Source: CAD feature listing. Evaluate the final solid. Frame: model axes, mm. Round coordinates to 2 decimals unless told otherwise and drop trailing zeros. Loops run counter-clockwise (first coordinate to the right, second up) from the corner with the lowest first, then second, coordinate; pieces in that order, holes last. Notation, with made-up numbers: M -27,-14.5 L 2,-14.5 A24 cw 2,10.5 Z; hole C -34,43.25 d11. An arc over 180 degrees is marked long. Answer as a JSON object with one key per item and string values.
from build123d import *

# Parameters (mm, degrees)
SKETCH1_R             = 5.75
BOSS_EXTRUDE1_DEPTH   = 3
BOSS_EXTRUDE2_DEPTH   = 0.15
CIRPATTERN1_COUNT     = 2
SKETCH4_R             = 2.5
CUT_EXTRUDE1_DEPTH    = 7.0000001
FILLET1_R             = 0.5
CHAMFER1_SIZE         = 1
CHAMFER1_SIZE2        = 1.191753593
CHAMFER1_PART_2_SIZE  = 1
CHAMFER1_PART_2_SIZE2 = 1.191753593


with BuildPart() as part:
    # Sketch1 → Boss-Extrude1 (new body, symmetric)
    with BuildSketch(Plane(origin=(0, 0, 0), x_dir=(1, 0, 0), z_dir=(0, 1, 0))):
        Circle(SKETCH1_R)
    extrude(amount=BOSS_EXTRUDE1_DEPTH, both=True)

    # Sketch3 → Boss-Extrude2 (add, symmetric)
    with BuildSketch(Plane(origin=(0, 0, 0), x_dir=(0.974370065, -0.224951054, 0), z_dir=(-0.224951054, -0.974370065, 0))):
        with BuildLine():
            Line((-3.7810451, 3.485569564), (-7.073832927, 7.724962303))
            Line((-7.073832927, 7.724962303), (-7.073832927, 60.5))
            ThreePointArc((-7.073832927, 60.5), (-6.19515327, 62.621320344), (-4.073832927, 63.5))
            Line((-4.073832927, 63.5), (-2.360798549, 63.5))
            ThreePointArc((-2.360798549, 63.5), (0.785773005, 62.385754426), (2.529923187, 59.539634982))
            add(Edge.make_bspline(
                [(5.379401291, 3.122506591), (7.423883814, 22.153749757), (6.457878795, 41.061478518), (2.529923187, 59.539634982)],
                knots=[0, 0, 0, 0, 0.933242383, 0.933242383, 0.933242383, 0.933242383], degree=3))
            add(Edge.make_bspline(
                [(5.379401291, 3.122506591), (1.050826141, 9.991793378), (-3.7810451, 3.485569564)],
                knots=[5.286447688, 5.286447688, 5.286447688, 7.20272538, 7.20272538, 7.20272538], degree=2, weights=[1, 0.575043633, 1]))
        make_face()
    boss_extrude2 = extrude(amount=BOSS_EXTRUDE2_DEPTH, both=True)

    # CirPattern1: Boss-Extrude2 ×2 about axis
    cirpattern1_axis = Axis((0, 3, 0), (0, -1, 0))
    for i in range(1, CIRPATTERN1_COUNT):
        add(boss_extrude2.rotate(cirpattern1_axis, i * 360 / CIRPATTERN1_COUNT))

    # Sketch4 → Cut-Extrude1 (cut, through all)
    with BuildSketch(Plane(origin=(0, 3, 0), x_dir=(1, 0, 0), z_dir=(0, 1, 0))):
        Circle(SKETCH4_R)
    extrude(amount=-CUT_EXTRUDE1_DEPTH, mode=Mode.SUBTRACT)

    # Fillet1
    fillet1_edges = [part.edges().sort_by_distance(p)[0] for p in [
        (-5.75, -3, 0),
        (-5.75, 3, 0),
    ]]
    fillet(fillet1_edges, radius=FILLET1_R)

    # Chamfer1
    chamfer1_edges = [part.edges().sort_by_distance(p)[0] for p in [
        (-2.5, -3, 0),
    ]]
    chamfer1_side = [part.faces().sort_by_distance(p)[0] for p in [
        (-2.5, 0, 0),
    ]]
    chamfer(chamfer1_edges, length=CHAMFER1_SIZE, length2=CHAMFER1_SIZE2, reference=chamfer1_side[0])

    # Chamfer1 part 2
    chamfer1_part_2_edges = [part.edges().sort_by_distance(p)[0] for p in [
        (-2.5, 3, 0),
    ]]
    chamfer1_part_2_side = [part.faces().sort_by_distance(p)[0] for p in [
        (-5.101507576, 3, 0),
    ]]
    chamfer(chamfer1_part_2_edges, length=CHAMFER1_PART_2_SIZE, length2=CHAMFER1_PART_2_SIZE2, reference=chamfer1_part_2_side[0])


solid = part.part
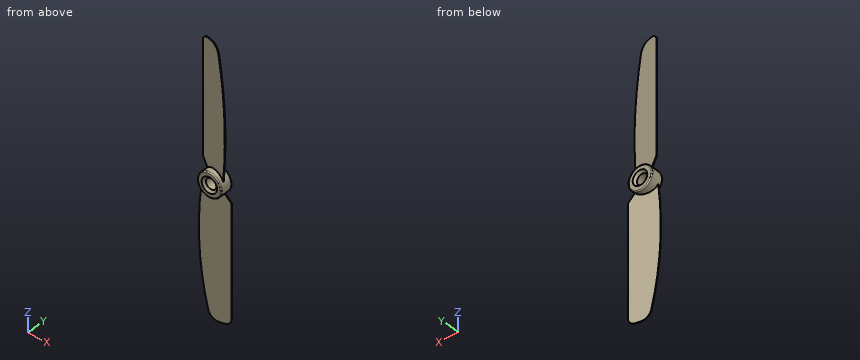
Item 1: Section A-A on z = 0. Return the cut outline in (x, y).
Answer sheet:
{"outline": "M -5.75,-2.5 A0.5 ccw -5.25,-3 L -3.69,-3 L -2.5,-2 L -2.5,1.81 L -3.5,3 L -5.25,3 A0.5 ccw -5.75,2.5 Z; M 2.5,-2 L 3.69,-3 L 5.25,-3 A0.5 ccw 5.75,-2.5 L 5.75,2.5 A0.5 ccw 5.25,3 L 3.5,3 L 2.5,1.81 Z"}
Item 2: Contact query for flat-ended pins moving along their axis: pin 1 Ø3 at (x, z) = (-5, -6.5) entering from +Y; pin 2 Ø6.5 at (x, z) = (0, 0) entering from +Y; pin 3 Ø1.5 at (x, z) = (2, -2) entering from -Y. Output: stop coordinate, or through.
Answer sheet:
{"pin 1": "stops at y = -0.65", "pin 2": "stops at y = 2.7", "pin 3": "stops at y = -2.9"}
Item 3: Line query: probe 1 along Z at (x, y) = (-0.5, 0.5); probe 2 along Z at (x, y) = (0.25, 1.5); probe 3 along X at (y, z) = (-0.85, 0). Output: solid intervals per line, ascending. Write a range as from..to.
Answer sheet:
{"probe 1": "z = -5.73..-2.45, 2.45..5.73", "probe 2": "z = -5.74..-2.49, 2.49..5.74", "probe 3": "x = -5.75..-2.5, 2.5..5.75"}
